Verification items for this drawing (mm, ordinates from the low corner). A direction names the side the tool comes from. Round coordinates to 2 decimals unless told otherwise and drop trailing zeros. Loops run counter-clockwise (first coordinate to the right, second up) from the corner with the lowest first, then second, coordinate; pieces in that order, holes last. Notation, with made-up numbers: (24.5, -29.5) - (78.5, -29.5) arc R5 ccw to (78.5, -25.5) - close; hole circle Ø10 at (-25, -14). An arc over 180 degrees is marked (long way). Answer in a Markdown table with one row per item. Add a question column.
(1) Cross-section at B-B on y = 28.25. Enter the section's corners in (x, z), then the cut area to 3 significant figures.
(2) Gauge pin test, flat ends, axial feed: pin 1 (1 mm diameter, centred on x = 10.5, y = 26.5, fed in from +Z); pin 2 (10 mm diameter, centred on x = 16.5, z = 8.5, fed in from -Y); pin 3 (10 mm diameter, centred on x = 29, y = 17.5, fed in from +Z); pin 4 (4.5 mm diameter, centred on x = 25.5, z = 12.5, fed in from -Y). Record the tip position at first contact, or that the pin passes through.
(3) Cross-section at A-A on z = 16.25. Enter the section's corners in (x, y).
(4) Cross-section at C-C on y = 4. Enter the section's corners in (x, z), then the cut area to 3 significant figures.
(5) Mould release check, pull along X, two halves, no side actions. Record for the marked faces 1, 2, 3 and 4: +X half, -X half, draft (parallel to the pull), parting line (faces both ways), or undercut.
(6) Cross-section at D-D on z = 6. Enter the section's corners in (x, y).
(7) Access from +Z, -Z, +X, -X, +Y, -Y to the whole of each face (thin tool, end or side, straight path). Record for the marked faces 5, 6, 7, 8 and 9.
(8) Thickness scan on line 1 along X through (y, z) = (1, 5); line 2 along X through (y, z) = (5, 16.25); line 3 along Y through (x, z) = (10.5, 1.25). Record the ranges inside material, lowest first.
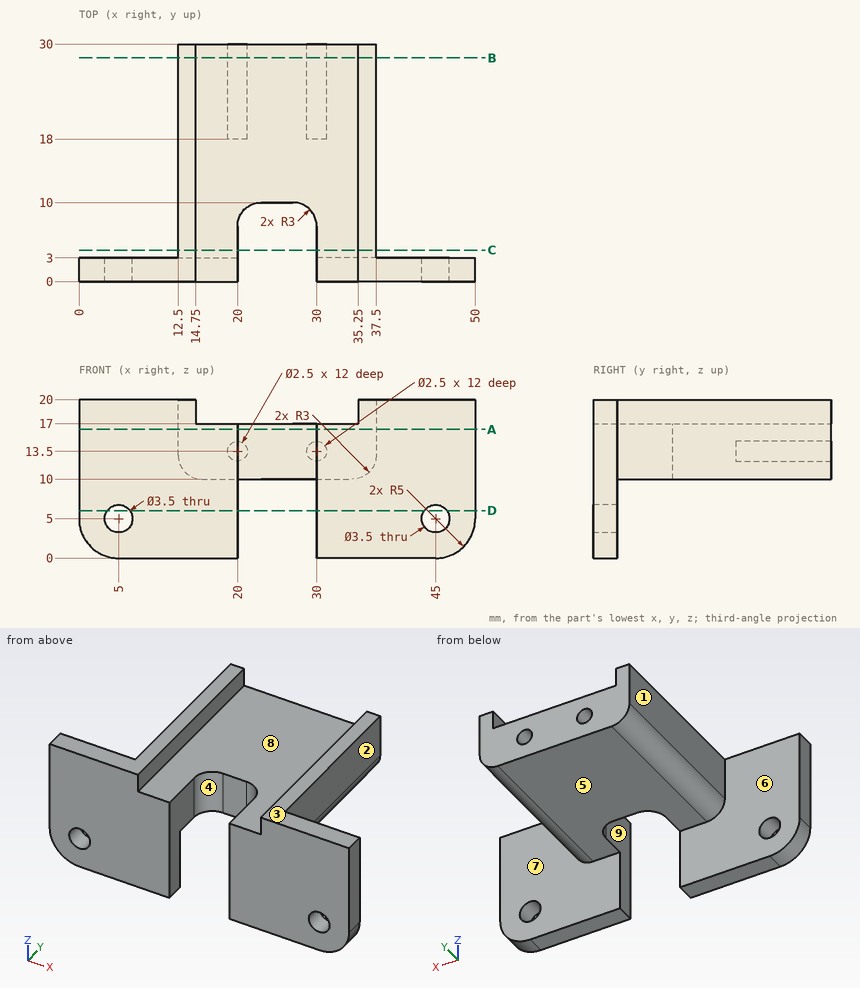
Answers:
| question | item | result |
|---|---|---|
| 1 | outline | (12.5, 13) arc R3 ccw to (15.5, 10) - (34.5, 10) arc R3 ccw to (37.5, 13) - (37.5, 20) - (35.25, 20) - (35.25, 17) - (14.75, 17) - (14.75, 20) - (12.5, 20) - close; hole circle Ø2.5 at (20, 13.5); hole circle Ø2.5 at (30, 13.5) |
| 1 | area | 175 mm^2 |
| 2 | pin 1 | passes through |
| 2 | pin 2 | stops at y = 0 |
| 2 | pin 3 | stops at z = 17 |
| 2 | pin 4 | stops at y = 9.9 |
| 3 | outline | (0, 0) - (20, 0) - (20, 7) arc R3 cw to (23, 10) - (27, 10) arc R3 cw to (30, 7) - (30, 0) - (50, 0) - (50, 3) - (37.5, 3) - (37.5, 30) - (12.5, 30) - (12.5, 3) - (0, 3) - close |
| 4 | outline | (12.5, 13) arc R3 ccw to (15.5, 10) - (20, 10) - (20, 17) - (14.75, 17) - (14.75, 20) - (12.5, 20) - close; (30, 10) - (34.5, 10) arc R3 ccw to (37.5, 13) - (37.5, 20) - (35.25, 20) - (35.25, 17) - (30, 17) - close |
| 4 | area | 115 mm^2 |
| 5 | face 1 | -X half |
| 5 | face 2 | +X half |
| 5 | face 3 | draft |
| 5 | face 4 | undercut |
| 6 | outline | (0, 0) - (3.56, 0) - (3.56, 3) - (0, 3) - close; (6.44, 0) - (20, 0) - (20, 3) - (6.44, 3) - close; (30, 0) - (43.56, 0) - (43.56, 3) - (30, 3) - close; (46.44, 0) - (50, 0) - (50, 3) - (46.44, 3) - close |
| 7 | face 5 | -Z, +X, -X, +Y |
| 7 | face 6 | -Z, -X, +Y |
| 7 | face 7 | -Z, +X, +Y |
| 7 | face 8 | +Z, +Y, -Y |
| 7 | face 9 | +Z, -Z, -Y |
| 8 | line 1 | x = 0 to 3.25, 6.75 to 20, 30 to 43.25, 46.75 to 50 |
| 8 | line 2 | x = 12.5 to 20, 30 to 37.5 |
| 8 | line 3 | y = 0 to 3 |
